from build123d import *

# Parameters (mm, degrees)
F0_R     = 11.049
F1_DEPTH = 7.0358


with BuildPart() as f1:
    # F0 (on Top) → F1 (new body)
    with BuildSketch(Plane.XY):
        with BuildLine():
            ThreePointArc((15.3606223584, -6.5915638429), (14.0515764921, -2.7419023957), (11.049, 0))
            ThreePointArc((11.049, 0), (7.8128228253, -7.8128228253), (0, -11.049))
            ThreePointArc((0, -11.049), (3.7722273632, -14.6239373815), (8.9372329685, -15.2006467181))
            ThreePointArc((8.9372329685, -15.2006467181), (11.4112106852, -10.3456815617), (15.3606223584, -6.5915638429))
        make_face()
        with BuildLine():
            ThreePointArc((0, 11.049), (7.8128228253, 7.8128228253), (11.049, 0))
            ThreePointArc((11.049, 0), (16.0517409884, 1.6673539034), (19.5923287649, 5.5752593056))
            ThreePointArc((19.5923287649, 5.5752593056), (19.648285181, 15.0586380241), (11.9809254143, 20.639784613))
            ThreePointArc((11.9809254143, 20.639784613), (7.1318081537, 17.0036295078), (1.2830021666, 15.4139658073))
            ThreePointArc((1.2830021666, 15.4139658073), (0.3997348377, 13.3025456864), (0, 11.049))
        make_face()
        with BuildLine():
            ThreePointArc((19.5923287649, 5.5752593056), (16.0517409884, 1.6673539034), (11.049, 0))
            ThreePointArc((11.049, 0), (14.0515764921, -2.7419023957), (15.3606223584, -6.5915638429))
            ThreePointArc((15.3606223584, -6.5915638429), (19.7194060635, -4.5374863882), (24.4904460645, -3.8626479736))
            ThreePointArc((24.4904460645, -3.8626479736), (24.4551845175, 2.1090263166), (19.5923287649, 5.5752593056))
        make_face()
        with BuildLine():
            ThreePointArc((-1.2878785477, 15.4227450117), (-0.401152017, 13.3073628417), (0, 11.049))
            ThreePointArc((0, 11.049), (0.3997348377, 13.3025456864), (1.2830021666, 15.4139658073))
            ThreePointArc((1.2830021666, 15.4139658073), (-0.0026133903, 15.367050345), (-1.2878785477, 15.4227450117))
        make_face()
        with BuildLine():
            ThreePointArc((-11.049, 0), (-7.8128228253, 7.8128228253), (0, 11.049))
            ThreePointArc((0, 11.049), (-0.401152017, 13.3073628417), (-1.2878785477, 15.4227450117))
            ThreePointArc((-1.2878785477, 15.4227450117), (-7.0848261597, 17.032079869), (-11.8887450472, 20.6538092378))
            ThreePointArc((-11.8887450472, 20.6538092378), (-19.6475824124, 15.060028688), (-19.5503933089, 5.4954851872))
            ThreePointArc((-19.5503933089, 5.4954851872), (-16.0139499505, 1.6428086369), (-11.049, 0))
        make_face()
        with BuildLine():
            ThreePointArc((-8.7698737274, -15.7762258045), (-3.5991350923, -14.870419784), (0, -11.049))
            ThreePointArc((0, -11.049), (-7.8128228253, -7.8128228253), (-11.049, 0))
            ThreePointArc((-11.049, 0), (-14.2101099006, -2.5648530064), (-15.7760277941, -6.3223771779))
            ThreePointArc((-15.7760277941, -6.3223771779), (-11.380052467, -10.3875833636), (-8.7698737274, -15.7762258045))
        make_face()
        with BuildLine():
            ThreePointArc((8.9372329685, -15.2006467181), (3.7722273632, -14.6239373815), (0, -11.049))
            ThreePointArc((0, -11.049), (-3.5991350923, -14.870419784), (-8.7698737274, -15.7762258045))
            ThreePointArc((-8.7698737274, -15.7762258045), (-8.5203506621, -16.839417556), (-8.3433460468, -17.9170574897))
            ThreePointArc((-8.3433460468, -17.9170574897), (-0.2261466235, -23.9881077254), (8.2807318523, -18.4763388586))
            ThreePointArc((8.2807318523, -18.4763388586), (8.523941199, -16.8214491689), (8.9372329685, -15.2006467181))
        make_face()
        with BuildLine():
            ThreePointArc((8.9372329685, -15.2006467181), (13.7625460617, -12.1000545802), (15.3606223584, -6.5915638429))
            ThreePointArc((15.3606223584, -6.5915638429), (11.4112106852, -10.3456815617), (8.9372329685, -15.2006467181))
        make_face()
        with BuildLine():
            ThreePointArc((24.4904460645, -3.8626479736), (20.5132557556, -7.1933790888), (15.3606223584, -6.5915638429))
            ThreePointArc((15.3606223584, -6.5915638429), (13.7625460617, -12.1000545802), (8.9372329685, -15.2006467181))
            ThreePointArc((8.9372329685, -15.2006467181), (8.7646746362, -16.8696960014), (8.2807318523, -18.4763388586))
            ThreePointArc((8.2807318523, -18.4763388586), (11.2032111335, -29.3509460419), (20.5279860839, -35.6633575195))
            ThreePointArc((20.5279860839, -35.6633575195), (31.2506997753, -34.5637006191), (38.8862682367, -26.9555517986))
            ThreePointArc((38.8862682367, -26.9555517986), (40.0671958518, -23.5618596089), (40.4674604904, -19.9909318682))
            ThreePointArc((40.4674604904, -19.9909318682), (35.7969947842, -8.6398687974), (24.4904460645, -3.8626479736))
        make_face()
        with Locations((24.3384604904, -19.9909318682)):
            Circle(F0_R, mode=Mode.SUBTRACT)
        with BuildLine():
            ThreePointArc((24.4904460645, -3.8626479736), (19.7194060635, -4.5374863882), (15.3606223584, -6.5915638429))
            ThreePointArc((15.3606223584, -6.5915638429), (20.5132557556, -7.1933790888), (24.4904460645, -3.8626479736))
        make_face()
        with BuildLine():
            ThreePointArc((-15.7760277941, -6.3223771779), (-14.2101099006, -2.5648530064), (-11.049, 0))
            ThreePointArc((-11.049, 0), (-16.0139499505, 1.6428086369), (-19.5503933089, 5.4954851872))
            ThreePointArc((-19.5503933089, 5.4954851872), (-25.2039351491, 2.4834340402), (-25.5915562379, -3.9106833611))
            ThreePointArc((-25.5915562379, -3.9106833611), (-20.4899973654, -4.3277912963), (-15.7760277941, -6.3223771779))
        make_face()
        with BuildLine():
            ThreePointArc((2.1504403371, 16.730865023), (1.6917102547, 16.0888900954), (1.2830021666, 15.4139658073))
            ThreePointArc((1.2830021666, 15.4139658073), (7.1318081537, 17.0036295078), (11.9809254143, 20.639784613))
            ThreePointArc((11.9809254143, 20.639784613), (6.5311461577, 20.0296234429), (2.1504403371, 16.730865023))
        make_face()
        with BuildLine():
            ThreePointArc((-1.2878785477, 15.4227450117), (-0.0026133903, 15.367050345), (1.2830021666, 15.4139658073))
            ThreePointArc((1.2830021666, 15.4139658073), (1.6917102547, 16.0888900954), (2.1504403371, 16.730865023))
            ThreePointArc((2.1504403371, 16.730865023), (-0.0310099814, 18.9779969426), (-2.0205494764, 16.5593072242))
            ThreePointArc((-2.0205494764, 16.5593072242), (-1.6357105315, 16.0029541604), (-1.2878785477, 15.4227450117))
        make_face()
        with BuildLine():
            ThreePointArc((-11.8887450472, 20.6538092378), (-7.0848261597, 17.032079869), (-1.2878785477, 15.4227450117))
            ThreePointArc((-1.2878785477, 15.4227450117), (-1.6357105315, 16.0029541604), (-2.0205494764, 16.5593072242))
            ThreePointArc((-2.0205494764, 16.5593072242), (-6.3882732082, 19.9715813543), (-11.8887450472, 20.6538092378))
        make_face()
        with BuildLine():
            ThreePointArc((8.2807318523, -18.4763388586), (8.7646746362, -16.8696960014), (8.9372329685, -15.2006467181))
            ThreePointArc((8.9372329685, -15.2006467181), (8.523941199, -16.8214491689), (8.2807318523, -18.4763388586))
        make_face()
        with BuildLine():
            ThreePointArc((-15.7760277941, -6.3223771779), (-14.2311309419, -12.5004895292), (-8.7698737274, -15.7762258045))
            ThreePointArc((-8.7698737274, -15.7762258045), (-11.380052467, -10.3875833636), (-15.7760277941, -6.3223771779))
        make_face()
        with BuildLine():
            ThreePointArc((-8.3433460468, -17.9170574897), (-8.6227516064, -16.8598193641), (-8.7698737274, -15.7762258045))
            ThreePointArc((-8.7698737274, -15.7762258045), (-14.2311309419, -12.5004895292), (-15.7760277941, -6.3223771779))
            ThreePointArc((-15.7760277941, -6.3223771779), (-21.2515182716, -7.4271607367), (-25.5915562379, -3.9106833611))
            ThreePointArc((-25.5915562379, -3.9106833611), (-36.4277245579, -9.3141188931), (-40.450284213, -20.7350940367))
            ThreePointArc((-40.450284213, -20.7350940367), (-35.3407505097, -31.7847546298), (-23.963299648, -36.1155681538))
            ThreePointArc((-23.963299648, -36.1155681538), (-12.8016582856, -31.2624373527), (-8.2094604904, -19.9909318682))
            ThreePointArc((-8.2094604904, -19.9909318682), (-8.2429666822, -18.9518360737), (-8.3433460468, -17.9170574897))
        make_face()
        with Locations((-24.3384604904, -19.9909318682)):
            Circle(F0_R, mode=Mode.SUBTRACT)
        with BuildLine():
            ThreePointArc((-8.3433460468, -17.9170574897), (-8.5203506621, -16.839417556), (-8.7698737274, -15.7762258045))
            ThreePointArc((-8.7698737274, -15.7762258045), (-8.6227516064, -16.8598193641), (-8.3433460468, -17.9170574897))
        make_face()
        with BuildLine():
            ThreePointArc((2.1504403371, 16.730865023), (6.5311461577, 20.0296234429), (11.9809254143, 20.639784613))
            ThreePointArc((11.9809254143, 20.639784613), (15.0947181843, 25.6757116075), (16.1814646071, 31.4959563034))
            ThreePointArc((16.1814646071, 31.4959563034), (14.0032432118, 39.5904246198), (8.0569166098, 45.4985770987))
            ThreePointArc((8.0569166098, 45.4985770987), (-0.1661064271, 47.6234752602), (-8.3285237566, 45.2765105392))
            ThreePointArc((-8.3285237566, 45.2765105392), (-15.9105328531, 33.804062255), (-11.8887450472, 20.6538092378))
            ThreePointArc((-11.8887450472, 20.6538092378), (-6.3882732082, 19.9715813543), (-2.0205494764, 16.5593072242))
            ThreePointArc((-2.0205494764, 16.5593072242), (-0.0310099814, 18.9779969426), (2.1504403371, 16.730865023))
        make_face()
        with Locations((0.0524646071, 31.4959563034)):
            Circle(F0_R, mode=Mode.SUBTRACT)
        with BuildLine():
            ThreePointArc((-25.5915562379, -3.9106833611), (-21.2515182716, -7.4271607367), (-15.7760277941, -6.3223771779))
            ThreePointArc((-15.7760277941, -6.3223771779), (-20.4899973654, -4.3277912963), (-25.5915562379, -3.9106833611))
        make_face()
        with BuildLine():
            Line((0, 52.0859286189), (-8.3285237566, 45.2765105392))
            ThreePointArc((-8.3285237566, 45.2765105392), (-0.1661064271, 47.6234752602), (8.0569166098, 45.4985770987))
            Line((8.0569166098, 45.4985770987), (0, 52.0859286189))
        make_face()
        with BuildLine():
            ThreePointArc((38.8862682367, -26.9555517986), (31.2506997753, -34.5637006191), (20.5279860839, -35.6633575195))
            Line((20.5279860839, -35.6633575195), (36.7174671022, -39.5995448364))
            Line((36.7174671022, -39.5995448364), (38.8862682367, -26.9555517986))
        make_face()
        with BuildLine():
            ThreePointArc((-23.963299648, -36.1155681538), (-35.3407505097, -31.7847546298), (-40.450284213, -20.7350940367))
            Line((-40.450284213, -20.7350940367), (-39.7229656538, -36.4822374832))
            Line((-39.7229656538, -36.4822374832), (-23.963299648, -36.1155681538))
        make_face()
    extrude(amount=F1_DEPTH)


solid = f1.part
Input: part model. Units: mm. Frame: model coordinates. A direction names the side the tool comes from. Give positions to 0.01 mm unless a question says otherwise; leave off trailing zeros. Order: outer loops, then holes, each group sorted by start corner. A loop starts at its lowest first (then second) coordinate and runs counter-clockwise, first axis right, second up. Notation, with made-up numbers: (0, 27.5) -> (34, 27.5) arc R19 ccw to (34, 52.5) -> close; hole circle Ø2 at (11.5, 67.5). An arc over 180 degrees is marked (long way). Use one line per item in the form item = value.
1) Section D-D, the plane x = -18.5. Return loops of the section in (y, z), and give its area (3 significant figures).
Response values:
outline = (-35.03, 0) -> (-29.37, 0) -> (-29.37, 7.04) -> (-35.03, 7.04) -> close; (-10.61, 0) -> (16.85, 0) -> (16.85, 7.04) -> (-10.61, 7.04) -> close
area = 233 mm^2
2) Section B-B, the plane y = 1. Return loops of the section in (x, z), and give its area (3 significant figures).
Response values:
outline = (-25.91, 0) -> (-11, 0) -> (-11, 7.04) -> (-25.91, 7.04) -> close; (11, 0) -> (24.91, 0) -> (24.91, 7.04) -> (11, 7.04) -> close
area = 203 mm^2
3) First-contact query: pin 1 Ø1 at (y, z) = (37, 1.5) entering from -X; pin 2 Ø1.5 at (y, z) = (41.5, 5.5) entering from -X; pin 3 Ø20 at (x, y) = (-24.34, -19.99) entering from +Z; pin 4 Ø10 at (x, y) = (-0.5, 11) entering from -Z. Flat tips, straight axial feed; report the tip coordinate or a pass-through.
Response values:
pin_1 = -15.28
pin_2 = -13.16
pin_3 = through
pin_4 = 0
4) Reachability of faces 1 (the flat face through (28.5, -37.6, 3.5)), 2 (the flat face through (-12, -4, 7.036)) from +Z, -Z, +X, -X, +Y, -Y: full face, straight path, thin tool, end or side. Return the list, or none.
Response values:
face_1 = +Z, -Z, -Y
face_2 = +Z, +X, -X, +Y, -Y
5) Section A-A, the plane z = 1.75. Return loops of the section in (x, y).
Response values:
outline = (-40.45, -20.74) -> (-39.72, -36.48) -> (-23.96, -36.12) arc R16.13 ccw to (-8.34, -17.92) arc R8.87 ccw to (8.28, -18.48) arc R16.13 ccw to (20.53, -35.66) -> (36.72, -39.6) -> (38.89, -26.96) arc R16.13 ccw to (24.49, -3.86) arc R6.56 ccw to (19.59, 5.58) arc R10.39 ccw to (11.98, 20.64) arc R16.13 ccw to (8.06, 45.5) -> (0, 52.09) -> (-8.33, 45.28) arc R16.13 ccw to (-11.89, 20.65) arc R10.39 ccw to (-19.55, 5.5) arc R6.56 ccw to (-25.59, -3.91) arc R16.13 ccw to start; hole circle Ø22.1 at (-24.34, -19.99); hole circle Ø22.1 at (0, 0); hole circle Ø22.1 at (0.05, 31.5); hole circle Ø22.1 at (24.34, -19.99)
6) Mould query, pull axis X, two halves, no side actions, for faces 3 (the flat face through (-12, -4, 0)), 4 (the flat face through (-40.09, -28.5, 3.47)), 5 (the cylindrical face through (-13.8, -16.67, 3.47)). Classes: pulls with the +X half, pulls with the -X half, needs draft (parallel to the pull), parting line crosses it, or undercut.
Response values:
face_3 = needs draft
face_4 = pulls with the -X half
face_5 = undercut
7) Line query: probe 1 along X at (y, z) = (-23, 5.75); probe 2 along Y at (x, z) = (5.5, 2.75); probe 3 along Y at (x, z) = (-7, 1). Output: solid intervals per line, ascending.
Response values:
probe_1 = -40.35 to -34.97, -13.71 to -8.49, -4.01 to 4.15, 8.49 to 13.71, 34.97 to 40.18
probe_2 = -22.14 to -9.58, 9.58 to 21.88, 41.11 to 47.59
probe_3 = -20.47 to -8.55, 8.55 to 22.99, 40 to 46.36
8) Section C-C, the plane x = 2. Return loops of the section in (y, z).
Response values:
outline = (-23.78, 0) -> (-10.87, 0) -> (-10.87, 7.04) -> (-23.78, 7.04) -> close; (10.87, 0) -> (20.62, 0) -> (20.62, 7.04) -> (10.87, 7.04) -> close; (42.37, 0) -> (50.45, 0) -> (50.45, 7.04) -> (42.37, 7.04) -> close
